Autodesk Inventor part; units mm, degrees
ref_plane "YZ Plane" through (0, 0, 0) normal (1, 0, 0) x (0, 1, 0)
ref_plane "XZ Plane" through (0, 0, 0) normal (0, 1, 0) x (-1, 0, 0)
ref_plane "XY Plane" through (0, 0, 0) normal (0, 0, 1) x (1, 0, 0)
sketch "Esboço1" plane through (0, 0, 0) normal (0, 1, 0) x (-1, 0, 0)
  line L0 (-48.4004, 17.271) -> (48.6103, 17.271)
  line L1 (48.6103, 17.271) -> (48.6103, -17.729)
  line L2 (48.6103, -17.729) -> (-48.4004, -17.729)
  line L3 (-48.4004, -17.729) -> (-48.4004, 17.271)
  line L4 (-51.9004, -19.229) -> (-51.9004, 19.271)
  line L5 (-51.9004, 19.271) -> (52.1103, 19.271)
  line L6 (-51.9004, -19.229) -> (52.1103, -19.229)
  line L7 (52.1103, -19.229) -> (52.1103, 19.271)
  circle A0 centre (-45.9004, 14.771) radius 1.75
  circle A1 centre (-45.9004, 14.771) radius 2.5
  circle A2 centre (-45.9004, -15.229) radius 1.75
  circle A3 centre (-45.9004, -15.229) radius 2.5
  circle A4 centre (46.1103, 14.771) radius 2.5
  circle A5 centre (46.1103, 14.771) radius 1.75
  circle A6 centre (46.1103, -15.229) radius 2.5
  circle A7 centre (46.1103, -15.229) radius 1.75
  line L8 (26.9024, 10.578) -> (26.9024, -11.7995)
  line L9 (-30.4004, -2.229) -> (-20.4004, -2.229)
  line L10 (-20.4004, -2.229) -> (-20.4004, -12.229)
  line L11 (-20.4004, -12.229) -> (-30.4004, -12.229)
  line L12 (-30.4004, -12.229) -> (-30.4004, -2.229)
  line L13 (-6.4004, 4.271) -> (-6.4004, -5.729)
  line L14 (-16.4004, 4.271) -> (-6.4004, 4.271)
  line L15 (-16.4004, -5.729) -> (-16.4004, 4.271)
  line L16 (-6.4004, -5.729) -> (-16.4004, -5.729)
  line L17 (-20.4004, 12.271) -> (-20.4004, 2.271)
  line L18 (-30.4004, 12.271) -> (-20.4004, 12.271)
  line L19 (-30.4004, 2.271) -> (-30.4004, 12.271)
  line L20 (-20.4004, 2.271) -> (-30.4004, 2.271)
  line L21 (-34.4004, 4.271) -> (-34.4004, -5.729)
  line L22 (-44.4004, 4.271) -> (-34.4004, 4.271)
  line L23 (-44.4004, -5.729) -> (-44.4004, 4.271)
  line L24 (-34.4004, -5.729) -> (-44.4004, -5.729)
  line L25 (31.4236, 11.771) -> (41.4236, 11.771)
  line L26 (41.4236, 11.771) -> (41.4236, -8.229)
  line L27 (41.4236, -8.229) -> (31.4236, -8.229)
  line L28 (31.4236, -8.229) -> (31.4236, 11.771)
  circle A8 centre (-25.4004, 7.271) radius 3.5
  circle A9 centre (-11.4004, -0.729) radius 3.5
  circle A10 centre (-25.4004, -7.729) radius 3.5
  circle A11 centre (-39.4004, -0.729) radius 3.5
  line L29 (-43.6091, 15.771) -> (43.819, 15.771)
  line L30 (-46.9004, -12.9377) -> (-46.9004, 12.4797)
  line L31 (43.819, -16.229) -> (-43.6091, -16.229)
  line L32 (47.1103, 12.4797) -> (47.1103, -12.9377)
  circle A12 centre (0.1524, 12.1393) radius 1.25
  circle A13 centre (25.6524, -13.3607) radius 1.25
  circle A14 centre (25.6524, 12.1393) radius 1.25
  circle A15 centre (0.1524, -13.3607) radius 1.25
  circle A16 centre (0.1524, -13.3607) radius 2
  circle A17 centre (0.1524, 12.1393) radius 2
  circle A18 centre (25.6524, 12.1393) radius 2
  circle A19 centre (25.6524, -13.3607) radius 2
  line L33 (3.9024, 13.3893) -> (21.9024, 13.3893)
  line L34 (21.9024, 13.3893) -> (21.9024, 6.3893)
  line L35 (21.9024, 6.3893) -> (3.9024, 6.3893)
  line L36 (3.9024, 6.3893) -> (3.9024, 13.3893)
  line L37 (-1.0976, -11.7995) -> (-1.0976, 10.578)
  line L38 (-1.0976, 12.1393) -> (-1.0976, 12.271)
  line L39 (1.7137, 13.3893) -> (24.0912, 13.3893)
  line L40 (26.9024, -14.6107) -> (25.6524, -14.6107)
  line L41 (24.0912, -14.6107) -> (1.7137, -14.6107)
  line L42 (0.1524, -14.6107) -> (-1.0976, -14.6107)
  line L43 (-1.0976, 9.3893) -> (26.9024, 9.3893)
  line L44 (26.9024, 9.3893) -> (26.9024, -10.6107)
  line L45 (26.9024, -10.6107) -> (-1.0976, -10.6107)
  line L46 (-1.0976, -10.6107) -> (-1.0976, 9.3893)
  point P0 (0, 0)
  point P1 (-4.4505, -19.229)
  point P2 (-25.4004, -2.229)
  point P3 (12.9024, 6.3893)
  point P4 (12.9024, 13.3893)
  point P5 (26.9024, -10.6107)
  point P6 (-1.0976, -10.6107)
  dimension "d35" = 2.5
  dimension "d36" = 2.5
  dimension "d38" = 2.5
  dimension "d0" = 3.5
  dimension "d1" = 2
  dimension "d2" = 3.5
  dimension "d3" = 3.5
  dimension "d4" = 5
  dimension "d5" = 3.5
  dimension "d6" = 5
  dimension "d7" = 5
  dimension "d8" = 3.5
  dimension "d9" = 5
  dimension "d10" = 3.5
  dimension "d11" = 104.0106
  dimension "d12" = 38.5
  dimension "d13" = 28
  dimension "d14" = 10
  dimension "d15" = 10
  dimension "d16" = 10
  dimension "d17" = 10
  dimension "d18" = 10
  dimension "d19" = 10
  dimension "d20" = 10
  dimension "d21" = 10
  dimension "d22" = 10
  dimension "d23" = 20
  dimension "d24" = 4
  dimension "d25" = 4
  dimension "d26" = 4
  dimension "d27" = 4
  dimension "d28" = 5.5
  dimension "d29" = 7
  dimension "d30" = 7
  dimension "d31" = 7
  dimension "d32" = 7
  dimension "d33" = 1.5
  dimension "d34" = 4.5
  dimension "d37" = 2.5
  dimension "d39" = 4
  dimension "d40" = 4
  dimension "d41" = 4
  dimension "d42" = 4
  dimension "d43" = 5
  dimension "d44" = 7
  dimension "d47" = 2.3817
  dimension "d48" = 28
  dimension "d49" = 4
  dimension "d50" = 4
extrude "Extrusão1" add sketch "Esboço1" along normal blind 2 contours L0 A1 L3 | L0 A4 L29 A1 | A1 | A1 L30 A3 L3 | L0 L1 A4 | A4 | A3 L2 L3 | A3 | L1 A6 L32 A4 | A3 L31 A6 L2 | A6 | L1 L2 A6
extrude "Extrusão2" add sketch "Esboço1" along normal blind 1 contours L29 A4 L32 A6 L31 A3 L30 A1 | L8 L43 L34 L39 A18 | A18 | L8 A19 L41 A16 L37 L45 | L43 L36 L33 L34 | A19 | L43 L37 A17 L39 L36 | A16 | A17 | L9 L10 L11 L12 | L13 L16 L15 L14 | L17 L20 L19 L18 | L21 L24 L23 L22 | A12 | A13 | A14 | A15
properties part number "tampa_lcd_botoes"
Here's how the part is built. I have some questions about the finished solid (model axes, mm). A direction names the side the tool comes from. Give positions to 0.01 mm unless a question says otherwise; leave off trailing zeros. Write each loop counter-clockwise with the first axis right and the second up, starting at its lowest first coordinate (ties: lowest second). Pieces come first, ordered by that corner, then holes. Notation, with made-up numbers: M 77,5.25 L 97,5.25 A13 ccw 97,16.25 Z; hole C 78.25,-1 d6. An arc over 180 degrees is marked long. Put each result on its own line as item: value. Start each with the question number.
Item 1: If we section it at D-D, the plane x = 10.5: Write out the boundary of the cut face in (y, z).
Item 2: On a 3-axis mill with a long thin cutter (end or side, diameter ignored), from which of +Z, -Z, +X, -X, +Y, -Y can I reach the whole of each face in a straight line? I mean faces 5 (the flat face through (11, 1, 4)), 6 (the cylindrical face through (44.23, 0.99, -15.75)). Say none if no direction works.
Item 3: Will this pin go through, and if not, where does the flat tip stop? pin 1 (16 mm diameter, centred on x = 17.5, z = 1.5, fed in from +Y).
Item 4: If we section it at C-C, the plane y = 1.7: Write out the boundary of the cut face in (x, z).
Item 5: Thinking about a two-plate mould opening in Z: for faces 1 (the flat face through (48.4, 1, 0)), 2 (the flat face through (1, 1, 17.271)), 3 (the flat face through (-1, 1, -17.729)), 4 (the cylindrical face through (44.284, 0.986, 15.441)), which applies, +Z half, -Z half, draft (parallel to the pull), parting line (faces both ways), or undercut?
Item 6: If we section it at A-A, the plane x = -4.5: Write out the boundary of the cut face in (y, z), then the cut area to 3 significant figures.
Item 7: If we section it at B-B, the plane x = -28.5: Write out the boundary of the cut face in (y, z), then the cut area to 3 significant figures.
Item 8: I need wall thicknesses on L1, parallel to Z at x = -17.5, y = 0.7; L2, parallel to Z at x = -38, y = 1.85; L3, parallel to X at y = 0.5, z = 15. Which ranges of each line are inside material? Lowest first, please. Write a range as from..to.
Values:
1. outline: M 0,-17.73 L 2,-17.73 L 2,-16.23 L 1,-16.23 L 1,-4.11 L 0,-4.11 Z; M 0,2.65 L 1,2.65 L 1,15.77 L 2,15.77 L 2,17.27 L 0,17.27 Z
2. face 5: +Y
2. face 6: +Y, -Y
3. pin 1: y = 1
4. outline: M -48.61,-17.73 L 48.4,-17.73 L 48.4,17.27 L -48.61,17.27 Z; hole C -46.11,-15.23 d3.5; hole C -46.11,14.77 d3.5; hole M -47.11,-12.94 A2.5 cw -43.82,-16.23 L 43.61,-16.23 A2.5 cw 46.9,-12.94 L 46.9,12.48 A2.5 cw 43.61,15.77 L -43.82,15.77 A2.5 cw -47.11,12.48 Z; hole C 45.9,-15.23 d3.5; hole C 45.9,14.77 d3.5
5. face 1: draft
5. face 2: +Z half
5. face 3: -Z half
5. face 4: undercut
6. outline: M 0,-17.73 L 2,-17.73 L 2,-16.23 L 1,-16.23 L 1,-10.61 L 0,-10.61 Z; M 0,9.39 L 1,9.39 L 1,15.77 L 2,15.77 L 2,17.27 L 0,17.27 Z
6. area: 18.0 mm²
7. outline: M 0,-17.73 L 2,-17.73 L 2,-16.23 L 1,-16.23 L 1,15.77 L 2,15.77 L 2,17.27 L 0,17.27 Z
7. area: 38.0 mm²
8. L1: -17.73..-10.61, 9.39..17.27
8. L2: -17.73..-16.23, 15.77..17.27
8. L3: -48.61..-47.85, -44.38..44.17, 47.64..48.4
